```python
from build123d import *

# Parameters (mm, degrees)
SCHIZZO2_W                   = 30
SCHIZZO2_H                   = 10
ESTRUSIONE_ESTRUSIONE1_DEPTH = 5
SCHIZZO3_W                   = 13
SCHIZZO3_H                   = 10
TAGLIO_ESTRUSIONE1_DEPTH     = 0.6
SMUSSO1_SIZE                 = 1


with BuildPart() as part:
    # Schizzo2 → Estrusione-Estrusione1 (new body)
    with BuildSketch(Plane.XY):
        Rectangle(SCHIZZO2_W, SCHIZZO2_H)
        with BuildLine():
            Line((-9, -1.75), (-11, -1.75))
            ThreePointArc((-11, -1.75), (-12.75, 0), (-11, 1.75))
            Line((-11, 1.75), (-9, 1.75))
            ThreePointArc((-9, 1.75), (-7.25, 0), (-9, -1.75))
        make_face(mode=Mode.SUBTRACT)
        with BuildLine():
            Line((9, -1.75), (11, -1.75))
            ThreePointArc((11, -1.75), (12.75, 0), (11, 1.75))
            Line((11, 1.75), (9, 1.75))
            ThreePointArc((9, 1.75), (7.25, 0), (9, -1.75))
        make_face(mode=Mode.SUBTRACT)
    extrude(amount=-ESTRUSIONE_ESTRUSIONE1_DEPTH)

    # Schizzo3 → Taglio-Estrusione1 (cut)
    with BuildSketch(Plane.XY):
        Rectangle(SCHIZZO3_W, SCHIZZO3_H)
    extrude(amount=-TAGLIO_ESTRUSIONE1_DEPTH, mode=Mode.SUBTRACT)

    # Smusso1
    smusso1_edges = [part.edges().sort_by_distance(p)[0] for p in [
        (-15, 5, -2.5),
        (15, 5, -2.5),
        (15, -5, -2.5),
        (-15, -5, -2.5),
    ]]
    chamfer(smusso1_edges, length=SMUSSO1_SIZE)


solid = part.part
```
Read the model definition and answer for the solid it produces. Units are mm, in the model's axes. A direction names the side the tool comes from. Round coordinates to 2 decimals unless told otherwise and drop trailing zeros. Write each loop counter-clockwise with the first axis right and the second up, starting at its lowest first coordinate (ties: lowest second). Pieces come first, ordered by that corner, then holes. Notation, with made-up numbers: (-13.75, -35.5) -> (1.25, -35.5) arc R6 cw to (1.25, -29.5) -> close; hole circle Ø2 at (84.25, 70.5). An arc over 180 degrees is marked (long way). Answer in a Markdown table with one row per item. Add a question column.
1) Find section B-B, the plane z = -2.35. Determine the outline of the cut face in (x, y), and give its area (3 significant figures).
2) Find section A-A, the plane y = 0. Determine the outline of the cut face in (x, z).
3) Consider line 1 (Y direction, x = 9.5, z = -1.15); line 2 (X direction, y = -0.5, z = -2.45); line 3 (Z direction, x = -5.5, y = 1.75). Determine where each line is inside the solid, lowest interval first.
4) Find section D-D, the plane x = -5. Determine the outline of the cut face in (y, z), and give its area (3 significant figures).
5) Find section C-C, the plane y = 2.75. Determine the outline of the cut face in (x, z).
6) Which of the six approach directions +Z, -Z, +X, -X, +Y, -Y give full straight-line access (tool end or side, diameter ignored) to faces 1 (the face through (0, 0, -0.6)), 2 (the face through (15, 0, -2)), 3 (the face through (-10, 1.75, -2))?
7) Given P1, Ø3, axis at x = 2.5, y = 1, coming from the +Z side, flat-ended and moving along its own axis, determine where the tip first touches the part or whether it passes through.
8) Determine the mould class of faces 4 (the face through (14.5, -4.5, -2.5)), 5 (the face through (12.75, -0.04, -2.46)), 6 (the face through (0, -5, -2)), 7 (the face through (-15, 0, -2)) for opening direction X: pulls with the +X half, pulls with the -X half, needs draft (parallel to the pull), parting line crosses it, or undercut.
Findings below:
| question | item | result |
|---|---|---|
| 1 | outline | (-15, -4) -> (-14, -5) -> (14, -5) -> (15, -4) -> (15, 4) -> (14, 5) -> (-14, 5) -> (-15, 4) -> close; hole (-11, -1.75) -> (-9, -1.75) arc R1.75 ccw to (-9, 1.75) -> (-11, 1.75) arc R1.75 ccw to start; hole (9, -1.75) -> (11, -1.75) arc R1.75 ccw to (11, 1.75) -> (9, 1.75) arc R1.75 ccw to start |
| 1 | area | 265 mm² |
| 2 | outline | (-15, -5) -> (-12.75, -5) -> (-12.75, 0) -> (-15, 0) -> close; (-7.25, -5) -> (7.25, -5) -> (7.25, 0) -> (6.5, 0) -> (6.5, -0.6) -> (-6.5, -0.6) -> (-6.5, 0) -> (-7.25, 0) -> close; (12.75, -5) -> (15, -5) -> (15, 0) -> (12.75, 0) -> close |
| 3 | line 1 | -5 to -1.75, 1.75 to 5 |
| 3 | line 2 | -15 to -12.68, -7.32 to 7.32, 12.68 to 15 |
| 3 | line 3 | -5 to -0.6 |
| 4 | outline | (-5, -5) -> (5, -5) -> (5, -0.6) -> (-5, -0.6) -> close |
| 4 | area | 44.0 mm² |
| 5 | outline | (-15, -5) -> (15, -5) -> (15, 0) -> (6.5, 0) -> (6.5, -0.6) -> (-6.5, -0.6) -> (-6.5, 0) -> (-15, 0) -> close |
| 6 | face 1 | +Z, +Y, -Y |
| 6 | face 2 | +Z, -Z, +X, +Y, -Y |
| 6 | face 3 | +Z, -Z |
| 7 | P1 | z = -0.6 |
| 8 | face 4 | pulls with the +X half |
| 8 | face 5 | undercut |
| 8 | face 6 | needs draft |
| 8 | face 7 | pulls with the -X half |
